Model file for the job. Use its own axes, mm. A direction names the side the tool comes from. Give positions to 0.01 mm unless a question says otherwise; leave off trailing zeros. Order: outer loops, then holes, each group sorted by start corner. A loop starts at its lowest first (then second) coordinate and runs counter-clockwise, first axis right, second up. Notation, with made-up numbers: M 54,10 L 104,10 A6 ccw 104,21 Z; hole C -39.5,-27 d4. An arc over 180 degrees is marked long. Return JSON: item names as keys, results as strings. Group by question number.
1. Slice it at D-D on y = -16. List the corners of the cut face in (x, z).
2. Slice it at A-A on y = 0. List the corners of the cut face in (x, z), then the cut area to 4 significant figures.
3. Wall check: probe 1 along Z at (x, y) = (2.1, 0); probe 2 along Y at (x, z) = (10.5, 7); probe 3 along Y at (x, z) = (21, 15.5). Give the ranges that are in metal, low to high. Write a range as [from, to].
4. Pin check, flat tips, straight feed: pin 1 (7 mm diameter, centred on x = 142, y = 0, fed in from -Z); pin 2 (4 mm diameter, centred on y = 16, z = 8, fed in from +X); pin 3 (1 mm diameter, centred on x = 52, y = 20, fed in from +Z) (3 decimals); pin 4 (5 mm diameter, centred on x = 86, y = 11, fed in from +Z). Stop position of each tip, or through.
5. Two-plate mould, pull along Y, no slides. Class faces 4 (the face through (74, -22.5, 8)), 5 (the face through (74, 0, -6)), 6 (the face through (78, 0, -4)): released by +Y, released by -Y, zero draft, split by the parting line, or undercut.
6. 3-axis set-ups, long thin cutter, end or side, ignore diameter. For faces 1 (the face through (74, 14, 0)), 2 (the face through (78, 3.5, -2)), 3 (the face through (1.48, 0.54, -3.44)): which of +Z, -Z, +X, -X, +Y, -Y reach the whole face in a straight line?
7. Slice it at B-B on z = 8. List the corners of the cut face in (x, y).
from build123d import *

# Parameters (mm, degrees)
F1_DEPTH = 150
F3_DEPTH = 147
F4_R     = 2.5
F5_DEPTH = 3
F6_R     = 1.5
F7_DEPTH = 3
F8_R     = 3
F9_DEPTH = 2


with BuildPart() as f1:
    # F0 (on Right) → F1 (new body)
    with BuildSketch(Plane.YZ):
        with BuildLine():
            Line((-22.5, 15), (-22.5, 0))
            Line((-22.5, 0), (-4.9, 0))
            Line((-4.9, 0), (-4.9, -6))
            Line((-4.9, -6), (4.9, -6))
            Line((4.9, -6), (4.9, 0))
            Line((4.9, 0), (22.5, 0))
            Line((22.5, 0), (22.5, 15))
            ThreePointArc((22.5, 15), (0, 37.5), (-22.5, 15))
        make_face()
    extrude(amount=F1_DEPTH)

    # F2 (on face) → F3 (cut)
    with BuildSketch(Plane.YZ.offset(150)):
        with BuildLine():
            Line((-19.5, 11), (-19.5, 1))
            Line((-19.5, 1), (-3.5, 1))
            Line((-3.5, 1), (-3.5, -4))
            Line((-3.5, -4), (3.5, -4))
            Line((3.5, -4), (3.5, 1))
            Line((3.5, 1), (19.5, 1))
            Line((19.5, 1), (19.5, 11))
            Line((19.5, 11), (21.5, 11))
            Line((21.5, 11), (21.5, 13))
            Line((21.5, 13), (19.5, 13))
            Line((19.5, 13), (19.5, 15))
            Line((19.5, 15), (21.5, 15))
            ThreePointArc((21.5, 15), (19.634412, 23.76013), (14.361407, 31))
            Line((14.361407, 31), (5.5, 17.678008))
            Line((5.5, 17.678008), (4.578571, 18.459456))
            Line((4.578571, 18.459456), (13.439978, 31.781448))
            ThreePointArc((13.439978, 31.781448), (0, 36.5), (-13.439978, 31.781448))
            Line((-13.439978, 31.781448), (-4.578571, 18.459456))
            Line((-4.578571, 18.459456), (-5.5, 17.678008))
            Line((-5.5, 17.678008), (-14.361407, 31))
            ThreePointArc((-14.361407, 31), (-19.634412, 23.76013), (-21.5, 15))
            Line((-21.5, 15), (-19.5, 15))
            Line((-19.5, 15), (-19.5, 13))
            Line((-19.5, 13), (-21.5, 13))
            Line((-21.5, 13), (-21.5, 11))
            Line((-21.5, 11), (-19.5, 11))
        make_face()
    extrude(amount=-F3_DEPTH, mode=Mode.SUBTRACT)

    # F4 (on face) → F5 (cut, through all)
    with BuildSketch(Plane(origin=(0, 0, 0), x_dir=(0, -1, 0), z_dir=(-1, 0, 0))):
        with Locations((0, -1)):
            Circle(F4_R)
    extrude(amount=-F5_DEPTH, mode=Mode.SUBTRACT)

    # F6 (on face) → F7 (cut, through all)
    with BuildSketch(Plane(origin=(0, 0, 0), x_dir=(0, -1, 0), z_dir=(-1, 0, 0))):
        with Locations((-16, 8)):
            Circle(F6_R)
        with Locations((-16, 17)):
            Circle(F6_R)
        with Locations((-8, 8)):
            Circle(F6_R)
        with Locations((-8, 17)):
            Circle(F6_R)
        with Locations((0, 8)):
            Circle(F6_R)
        with Locations((0, 17)):
            Circle(F6_R)
        with Locations((8, 8)):
            Circle(F6_R)
        with Locations((8, 17)):
            Circle(F6_R)
        with Locations((16, 8)):
            Circle(F6_R)
        with Locations((16, 17)):
            Circle(F6_R)
    extrude(amount=-F7_DEPTH, mode=Mode.SUBTRACT)

    # F8 (on face) → F9 (cut, through all)
    with BuildSketch(Plane(origin=(0, 0, -6), x_dir=(1, 0, 0), z_dir=(0, 0, -1))):
        with Locations((142, 0)):
            Circle(F8_R)
    extrude(amount=-F9_DEPTH, mode=Mode.SUBTRACT)


solid = f1.part
Result:
{
 "1": {"outline": "M 0,0 L 150,0 L 150,1 L 3,1 L 3,6.5 L 0,6.5 Z; M 0,9.5 L 3,9.5 L 3,15.5 L 0,15.5 Z; M 0,18.5 L 3,18.5 L 3,29.36 L 150,29.36 L 150,30.82 L 0,30.82 Z"},
 "2": {"outline": "M 0,-6 L 139,-6 L 139,-4 L 3,-4 L 3,-3.5 L 0,-3.5 Z; M 0,1.5 L 3,1.5 L 3,6.5 L 0,6.5 Z; M 0,9.5 L 3,9.5 L 3,15.5 L 0,15.5 Z; M 0,18.5 L 3,18.5 L 3,36.5 L 150,36.5 L 150,37.5 L 0,37.5 Z; M 145,-6 L 150,-6 L 150,-4 L 145,-4 Z", "area": "526.5 mm2"},
 "3": {"probe 1": "z = [-6, -3.5], [1.5, 6.5], [9.5, 15.5], [18.5, 37.5]", "probe 2": "y = [-22.5, -19.5], [19.5, 22.5]", "probe 3": "y = [-22.49, -21.49], [21.49, 22.49]"},
 "4": {"pin 1": "stops at z = -6", "pin 2": "stops at x = 3", "pin 3": "stops at z = 26.225", "pin 4": "stops at z = 35.83"},
 "5": {"face 4": "released by -Y", "face 5": "zero draft", "face 6": "undercut"},
 "6": {"face 1": "-Z, +X, -X, +Y", "face 2": "+X", "face 3": "+X, -X"},
 "7": {"outline": "M 0,-22.5 L 150,-22.5 L 150,-19.5 L 3,-19.5 L 3,-17.5 L 0,-17.5 Z; M 0,-14.5 L 3,-14.5 L 3,-9.5 L 0,-9.5 Z; M 0,-6.5 L 3,-6.5 L 3,-1.5 L 0,-1.5 Z; M 0,1.5 L 3,1.5 L 3,6.5 L 0,6.5 Z; M 0,9.5 L 3,9.5 L 3,14.5 L 0,14.5 Z; M 0,17.5 L 3,17.5 L 3,19.5 L 150,19.5 L 150,22.5 L 0,22.5 Z"}
}
